Geometry: final body of the model. Coordinates: model frame, mm. A direction names the side the tool comes from. Round coordinates to 2 decimals unless told otherwise and drop trailing zeros. Order: outer loops, then holes, each group sorted by start corner. A loop starts at its lowest first (then second) coordinate and runs counter-clockwise, first axis right, second up. Notation, with made-up numbers: (60.25, -27) - (90.25, -27) arc R18 cw to (90.25, -18) - close; hole circle Ø5 at (-31, 30). An arc over 180 degrees is marked (long way). Put each result on its own line as item: value. Start each with the question number.
(1) Material intervals for L1, parallel to X at y = -9, z = 17.5; L2, parallel to Y at x = -0.5, z = -7; L3, parallel to Y at x = -10, z = -2.5, sorted ascending. Write a range as [from, to].
(2) Pin query (flat end, axial travel): P1, Ø3, axis at y = -1, z = -1, coming from the -X side; P2, Ø6, axis at y = -5.5, z = -10.5, coming from the -X side; P3, Ø3, axis at y = -5.5, z = -15.5, coming from the -X side; P4, Ø4.5, axis at y = -7, z = 14.5, coming from the +X side. Return the tip coordinate at first contact, or that it passes through.
(3) Section A-A (y = -5.5). Output: boundary loops of the cut face in (x, z), and give its area (3 significant figures).
(4) Section C-C (z = -18). Output: boundary loops of the cut face in (x, y), and give its area (3 significant figures).
(5) Access query for faces 1 (the face through (-3.5, -9, -16)), 2 (the face through (-8, 10, 0)), 3 (the face through (3.5, -9, 16)), 4 (the face through (-10.7, 0.7, -3.6)), 5 (the face through (14, -9, -7.3)). Directions: +Z, -Z, +X, -X, +Y, -Y. A direction counts if a zero-diameter tool reaches every point of the face in a straight line with its end or side. Return the directions, or none.
(6) Section B-B (z = 0). Output: boundary loops of the cut face in (x, y).
(7) Section D-D (x = -7). Output: boundary loops of the cut face in (y, z).
(8) Pull-direction query (Z, two-part tool) for faces 6 (the face through (17, -9, 0)), 7 (the face through (-0.8, -9.37, 19.44)), 8 (the face through (-14, -9, 0)); classes: released by +Z, released by -Z, zero draft, split by the parting line, or undercut.
from build123d import *

# Parameters (mm, degrees)
SKETCH1_R           = 14
SKETCH1_R_2         = 2.1
SKETCH1_W           = 5.05387092
SKETCH1_H           = 14.6
BOSS_EXTRUDE1_DEPTH = 19
SKETCH2_R           = 4.5
BOSS_EXTRUDE2_DEPTH = 1.5
SKETCH3_R           = 2.5
BOSS_EXTRUDE3_DEPTH = 8.5


with BuildPart() as part:
    # Sketch1 → Boss-Extrude1 (new body)
    # profile 1 of 3: a face of its own
    with BuildSketch(Plane(origin=(0, 0, 0), x_dir=(1, 0, 0), z_dir=(0, 1, 0))):
        Circle(SKETCH1_R)
    # profile 2 of 3: a face of its own
    with BuildSketch(Plane(origin=(0, 0, 0), x_dir=(1, 0, 0), z_dir=(0, 1, 0))):
        with BuildLine():
            Line((-3.5, -17.5), (-3.5, 17.5))
            ThreePointArc((-3.5, 17.5), (0, 21), (3.5, 17.5))
            Line((3.5, 17.5), (3.5, -17.5))
            ThreePointArc((3.5, -17.5), (0, -21), (-3.5, -17.5))
        make_face()
        with Locations(Location((0, -17.5, 0), (0, 0, 270))):
            Circle(SKETCH1_R_2, mode=Mode.SUBTRACT)
        with Locations(Location((0, 17.5, 0), (0, 0, 270))):
            Circle(SKETCH1_R_2, mode=Mode.SUBTRACT)
    # profile 3 of 3: a face of its own
    with BuildSketch(Plane(origin=(0, 0, 0), x_dir=(1, 0, 0), z_dir=(0, 1, 0))):
        with Locations((14.47306454, 0)):
            Rectangle(SKETCH1_W, SKETCH1_H)
    extrude(amount=-BOSS_EXTRUDE1_DEPTH)

    # Sketch2 → Boss-Extrude2 (add)
    with BuildSketch(Plane(origin=(0, 0, 0), x_dir=(1, 0, 0), z_dir=(0, 1, 0))):
        with Locations(Location((-8, 0, 0), (0, 0, 270))):
            Circle(SKETCH2_R)
    extrude(amount=BOSS_EXTRUDE2_DEPTH)

    # Sketch3 → Boss-Extrude3 (add)
    with BuildSketch(Plane(origin=(0, 1.5, 0), x_dir=(1, 0, 0), z_dir=(0, 1, 0))):
        with Locations(Location((-8, 0, 0), (0, 0, 270))):
            Circle(SKETCH3_R)
    extrude(amount=BOSS_EXTRUDE3_DEPTH)


solid = part.part
Checks:
1. L1: x = [-3.5, -2.1], [2.1, 3.5]
1. L2: y = [-19, 0]
1. L3: y = [-19, 1.5]
2. P1: stops at x = -14
2. P2: stops at x = -11.82
2. P3: stops at x = -3.5
2. P4: stops at x = 6.78
3. outline: (-3.5, -17.5) arc R3.5 ccw to (3.5, -17.5) - (3.5, -13.56) arc R14 ccw to (11.95, -7.3) - (17, -7.3) - (17, 7.3) - (11.95, 7.3) arc R14 ccw to (3.5, 13.56) - (3.5, 17.5) arc R3.5 ccw to (-3.5, 17.5) - (-3.5, 13.56) arc R14 ccw to (-3.5, -13.56) - close; hole circle Ø4.2 at (0, -17.5); hole circle Ø4.2 at (0, 17.5)
3. area: 731 mm²
4. outline: (-3.46, -19) - (-2.04, -19) - (-2.04, 0) - (-3.46, 0) - close; (2.04, -19) - (3.46, -19) - (3.46, 0) - (2.04, 0) - close
4. area: 54.1 mm²
5. face 1: -Z, -X, +Y, -Y
5. face 2: +Z, -Z, +X, -X, +Y
5. face 3: +Z, +X, +Y, -Y
5. face 4: +Y
5. face 5: -Z, +X, +Y, -Y
6. outline: (-14, -19) - (17, -19) - (17, 0) - (-3.5, 0) - (-3.5, 1.5) - (-5.5, 1.5) - (-5.5, 10) - (-10.5, 10) - (-10.5, 1.5) - (-12.5, 1.5) - (-12.5, 0) - (-14, 0) - close
7. outline: (-19, -12.12) - (0, -12.12) - (0, -4.39) - (1.5, -4.39) - (1.5, -2.29) - (10, -2.29) - (10, 2.29) - (1.5, 2.29) - (1.5, 4.39) - (0, 4.39) - (0, 12.12) - (-19, 12.12) - close
8. face 6: zero draft
8. face 7: undercut
8. face 8: split by the parting line
